Can you work these out from the model? Positions are in its coordinate system, mm. Face numbers are marked on the shaded views. A direction names the side the tool comes from. Round coordinates to 2 decimals unless told otherwise and drop trailing zeros. Order: outer loops, then holes, each group sorted by start corner. A loop starts at its lowest first (then second) coordinate and runs counter-clockwise, first axis right, second up. Notation, with made-up numbers: M -26,46.5 L -19,46.5 A20 ccw -19,84.5 Z; hole C 21.25,35.25 d7. An arc over 180 degrees is marked long. Answer as a JSON object with one key per item and string values. Group by question number.
Autodesk Fusion 360 part; units mm, degrees
sketch "Sketch1" plane through (0, 0, 0) normal (0, 1, 0) x (1, 0, 0)
  circle A0 centre (0, 0) radius 19.05
  dimension "d1" = 38.1
extrude "Extrude1" add sketch "Sketch1" along normal blind 25.4 makes body 1
sketch "Sketch2" plane through (0, 25.4, 0) normal (0, 1, 0) x (-1, 0, 0)
  circle A0 centre (0, 0) radius 19.05
  circle A1 centre (0, 0) radius 12.7
  circle A2 centre (0, 0) radius 15.875
  dimension "d4" = 25.4
  dimension "d5" = 31.75
extrude "Extrude2" cut sketch "Sketch2" against normal blind 22.225 contours A2 bodies 1
sketch "Sketch3" plane through (0, 0, 0) normal (0, -1, 0) x (1, 0, 0)
  circle A0 centre (0, 0) radius 19.05
  line L0 (6.35, 3.6662) -> (0, 7.3323)
  line L1 (0, 7.3323) -> (-6.35, 3.6662)
  line L2 (-6.35, 3.6662) -> (-6.35, -3.6662)
  line L3 (-6.35, -3.6662) -> (0, -7.3323)
  line L4 (0, -7.3323) -> (6.35, -3.6662)
  line L5 (6.35, -3.6662) -> (6.35, 3.6662)
  line L6 (-11.43, 6.5991) -> (-11.43, -6.5991)
  line L7 (-11.43, -6.5991) -> (0, -13.1982)
  line L8 (0, -13.1982) -> (11.43, -6.5991)
  line L9 (11.43, -6.5991) -> (11.43, 6.5991)
  line L10 (11.43, 6.5991) -> (0, 13.1982)
  line L11 (0, 13.1982) -> (-11.43, 6.5991)
  dimension "d9" = 6.35
  dimension "d17" = 5.08
copy_body "Body->Comp1" bodies 1 removing the originals makes body 2 in component "Component"
extrude "Extrude1'" add sketch "Sketch3" along normal blind 3.175 contours L6 L7 L8 L9 L10 L11 bodies 2 in component "Component"
fillet "Fillet1" radius 5.08 1 edges at (-17.7608, 0, 6.8888) on bodies 2 in component "Component"
fillet "Fillet2" radius 2.54 6 edges at (-5.715, -3.175, 9.8987) (-11.43, -3.175, 0) (-5.715, -3.175, -9.8987) (5.715, -3.175, -9.8987) (5.715, -3.175, 9.8987) (11.43, -3.175, 0) on bodies 2 in component "Component"
sketch "Sketch4" plane through (0, 0, 0) normal (0, 1, 0) x (1, 0, 0)
  line L0 (6.35, 3.6662) -> (0, 7.3323)
  line L1 (0, 7.3323) -> (-6.35, 3.6662)
  line L2 (-6.35, 3.6662) -> (-6.35, -3.6662)
  line L3 (-6.35, -3.6662) -> (0, -7.3323)
  line L4 (0, -7.3323) -> (6.35, -3.6662)
  line L5 (6.35, -3.6662) -> (6.35, 3.6662)
  dimension "d27" = 6.35
extrude "Extrude2'" cut sketch "Sketch4" along normal blind 25.4 bodies 2 in component "Component"
component "Component" placed x (1, 0, 0) y (0, 1, 0) z (0, 0, 1) at (0, 0, 0)
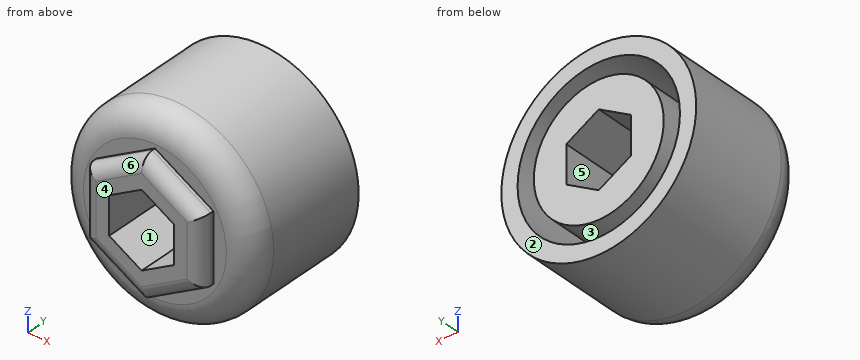
Item 1: If we mould it in two halves opening along Z, with no side actions, what happens to the marked faces 4, 5 and 6? For each: +Z half, -Z half, draft (parallel to the pull), parting line (faces both ways), or undercut.
Item 2: Suppose I cut it at B-B, the plane z = 0. Write out the boundary of the cut face in (x, y) (3 decimals).
Item 3: I'm going to push flat-ended pins straight in: pin 1 Ø3 at (x, z) = (1, -4) entering from -Y; pin 2 Ø6 at (y, z) = (10, 1.5) entering from -X; pin 3 Ø12 at (y, z) = (14.5, -13) entering from +X; pin 4 Ø5 at (y, z) = (14.5, -4) entering from +X. Where does each tip first touch, or does it pass through?
Item 4: On a 3-axis mill with a long thin cutter (end or side, diameter ignored), from which of +Z, -Z, +X, -X, +Y, -Y can I reach the whole of each face in a straight line? I mean the marked faces 1, 2 and 3. Say none if no direction works.
Item 5: I need wall thicknesses on line 1 (Z direction, x = 0, y = 16.75) (3 decimals); line 2 (X direction, y = 18, z = 1); line 3 (Z direction, x = 3, y = 14). Which ranges of each line are inside material? Lowest first, please.
Item 6: Suppose I cut it at A-A, the plane y = 12.5. Write out the boundary of the cut face in (x, z) (3 decimals), and give its area (3 significant figures).
Item 7: Suppose I cut it at C-C, the plane y = 1.25. Write out the boundary of the cut face in (x, z).
Computed:
{
 "1": {"face 4": "draft", "face 5": "undercut", "face 6": "+Z half"},
 "2": {"outline": "M -19.05,5.08 A5.08 ccw -13.97,0 L -11.43,0 L -11.43,-0.635 A2.54 ccw -8.89,-3.175 L -6.35,-3.175 L -6.35,25.4 L -12.7,25.4 L -12.7,3.175 L -15.875,3.175 L -15.875,25.4 L -19.05,25.4 Z; M 6.35,-3.175 L 8.89,-3.175 A2.54 ccw 11.43,-0.635 L 11.43,0 L 13.97,0 A5.08 ccw 19.05,5.08 L 19.05,25.4 L 15.875,25.4 L 15.875,3.175 L 12.7,3.175 L 12.7,25.4 L 6.35,25.4 Z"},
 "3": {"pin 1": "passes through", "pin 2": "stops at x = -19.05", "pin 3": "stops at x = 17.72", "pin 4": "stops at x = 18.99"},
 "4": {"face 1": "+Y, -Y", "face 2": "+Z, -Z, +X, -X, +Y", "face 3": "+Y"},
 "5": {"line 1": "z = -19.05 to -15.875, -12.7 to -7.332, 7.332 to 12.7, 15.875 to 19.05", "line 2": "x = -19.02 to -15.84, -12.66 to -6.35, 6.35 to 12.66, 15.84 to 19.02", "line 3": "z = -18.81 to -15.59, -12.34 to -5.6, 5.6 to 12.34, 15.59 to 18.81"},
 "6": {"outline": "C 0,0 d38.1; C 0,0 d25.4; hole C 0,0 d31.75; hole M -6.35,-3.666 L 0,-7.332 L 6.35,-3.666 L 6.35,3.666 L 0,7.332 L -6.35,3.666 Z", "area": "715 mm^2"},
 "7": {"outline": "C 0,0 d34.61; hole M -6.35,-3.67 L 0,-7.33 L 6.35,-3.67 L 6.35,3.67 L 0,7.33 L -6.35,3.67 Z"}
}
